```python
from build123d import *

# Parameters (mm, degrees)
SKICA2_W                 = 150
SKICA2_H                 = 4.2
SKICA2_W_2               = 18
SKICA2_H_2               = 1
P_IDAT_VYSUNUT_M2_DEPTH  = 0.4
SKICA3_R                 = 1.5
SKICA3_R_2               = 1.75
P_IDAT_VYSUNUT_M3_DEPTH  = 2.2
SKICA5_R                 = 1.9
P_IDAT_VYSUNUT_M5_DEPTH  = 2
ZKOSEN_2_SIZE            = 1.5
SKICA7_W                 = 1
SKICA7_H                 = 5
ODEBRAT_VYSUNUT_M1_DEPTH = 4


with BuildPart() as part:
    # Skica2 → Přidat vysunutím2 (new body)
    with BuildSketch(Plane.XY):
        Rectangle(SKICA2_W, SKICA2_H)
        with Locations((-5, -0.2)):
            Rectangle(SKICA2_W_2, SKICA2_H_2, mode=Mode.SUBTRACT)
    extrude(amount=P_IDAT_VYSUNUT_M2_DEPTH)

    # Skica3 → Přidat vysunutím3 (add)
    with BuildSketch(Plane.XY.offset(0.4)):
        with Locations((-50, -0.2)):
            Circle(SKICA3_R)
        with Locations((50, 0)):
            Circle(SKICA3_R_2)
    extrude(amount=P_IDAT_VYSUNUT_M3_DEPTH)

    # Skica5 → Přidat vysunutím5 (add)
    with BuildSketch(Plane.XY.offset(2.6)):
        with Locations((-50, -0.2)):
            Circle(SKICA5_R)
        with Locations((50, 0)):
            Circle(SKICA5_R)
    extrude(amount=P_IDAT_VYSUNUT_M5_DEPTH)

    # Zkosení2
    zkosen_2_edges = [part.edges().sort_by_distance(p)[0] for p in [
        (-51.9, -0.2, 4.6),
        (48.1, 0, 4.6),
    ]]
    chamfer(zkosen_2_edges, length=ZKOSEN_2_SIZE)

    # Skica7 → Odebrat vysunutím1 (cut)
    with BuildSketch(Plane.XY.offset(4.6)):
        with Locations((-50, -0.2)):
            Rectangle(SKICA7_W, SKICA7_H)
        with Locations((50, 0)):
            Rectangle(SKICA7_W, SKICA7_H)
    extrude(amount=-ODEBRAT_VYSUNUT_M1_DEPTH, mode=Mode.SUBTRACT)


solid = part.part
```
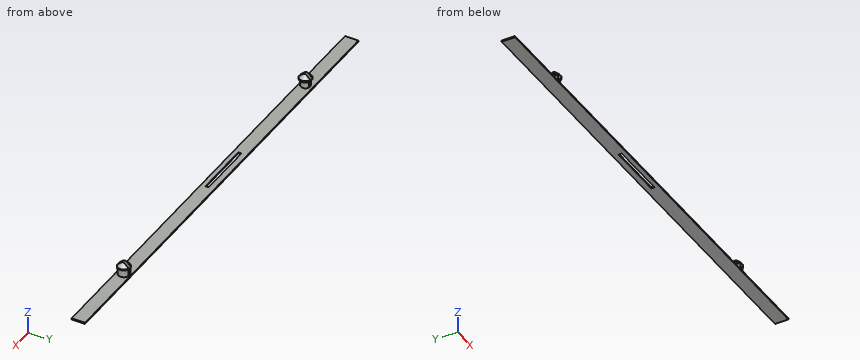
Check sheet for the modelled part. Datum: model origin and axes. Units: mm. Round coordinates to 2 decimals unless told otherwise and drop trailing zeros. Write each loop counter-clockwise with the first axis right and the second up, starting at its lowest first coordinate (ties: lowest second). Pieces come first, ordered by that corner, then holes. Notation, with made-up numbers: (52, -5.75) -> (84, -5.75) arc R21 ccw to (84, 27.25) -> close; hole circle Ø5 at (21.5, 15). An arc over 180 degrees is marked (long way). One line per question, with ' | ' between items. Start each with the question number.
1. Depth check by flat-ended pin: pin 1 (1.1 mm diameter, centred on y = 0.5, z = 3, fed in from +X); pin 2 (1.8 mm diameter, centred on y = -1, z = 2, fed in from -X). Enter the tip coordinate at first touch or a pass-through.
2. Sectioned sample at B-B, the plane z = 1.5. Record the cut outline in (x, y), then the cut area to 3 significant figures.
3. Scan lines: line 1 along X through (y, z) = (-0.2, 2); line 2 along X through (y, z) = (0.9, 2.05); line 3 along Z through (x, y) = (-28, -1.25). Record each from-to range of solid material in increasing order. Write a range as from..to.
4. Sectioned sample at C-C, the plane x = 38.5. Record the cut outline in (y, z).
5. Sectioned sample at A-A, the plane x = 1.5. Record the cut outline in (y, z).
Taken from the geometry:
1) pin 1: stops at x = 51.9 | pin 2: stops at x = -51.9
2) outline: (-50.5, -1.61) -> (-50.5, 1.21) arc R1.5 ccw to start; (-49.5, -1.61) arc R1.5 ccw to (-49.5, 1.21) -> close; (49.5, -1.68) -> (49.5, 1.68) arc R1.75 ccw to start; (50.5, -1.68) arc R1.75 ccw to (50.5, 1.68) -> close | area: 10.3 mm^2
3) line 1: x = -51.5..-50.5, -49.5..-48.5, 48.26..49.5, 50.5..51.74 | line 2: x = -51.02..-50.5, -49.5..-48.98, 48.5..49.5, 50.5..51.5 | line 3: z = 0..0.4
4) outline: (-2.1, 0) -> (2.1, 0) -> (2.1, 0.4) -> (-2.1, 0.4) -> close
5) outline: (-2.1, 0) -> (-0.7, 0) -> (-0.7, 0.4) -> (-2.1, 0.4) -> close; (0.3, 0) -> (2.1, 0) -> (2.1, 0.4) -> (0.3, 0.4) -> close
